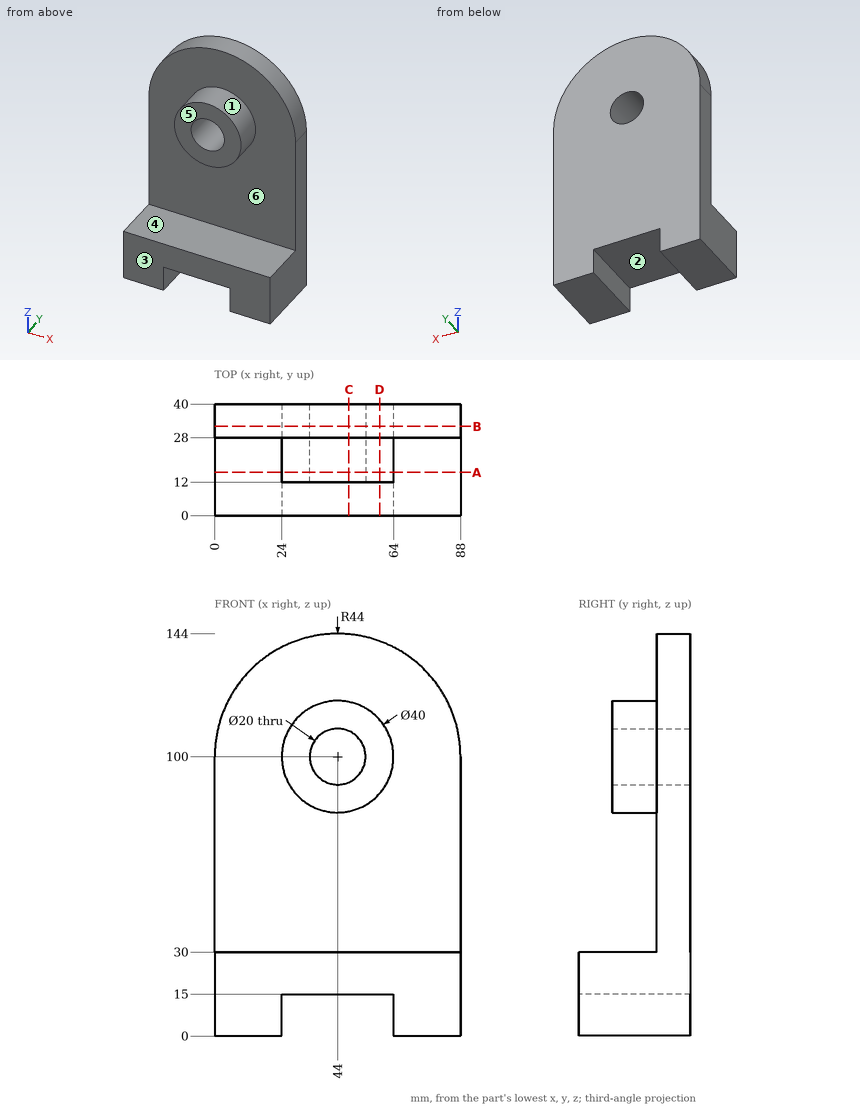
Answer from the drawing. Dimensions are ordinates in mm from the lowest x, y and z of the part. A direction names the side the tool comes from. Round coordinates to 2 decimals unless told otherwise and drop trailing zeros. Write each loop counter-clockwise with the first axis right and the second up, starting at its lowest first coordinate (ties: lowest second). Pieces come first, ordered by that corner, then holes. Notation, with made-up numbers: M 25.5,69.25 L 58.5,69.25 A16 ccw 58.5,85.25 Z; hole C 87,10 d8. An arc over 180 degrees is marked long. One line per item, written item: value.
Q1. Find section D-D on x = 59. Write down the section's boundary in (y, z), plus the area to 3 significant figures.
Data:
outline: M 0,15 L 40,15 L 40,141.36 L 28,141.36 L 28,113.23 L 12,113.23 L 12,86.77 L 28,86.77 L 28,30 L 0,30 Z
area: 2,360 mm2
Q2. Find section C-C on x = 48. Write down the section's boundary in (y, z), plus the area to 3 significant figures.
Data:
outline: M 0,15 L 40,15 L 40,90.83 L 12,90.83 L 12,80.4 L 28,80.4 L 28,30 L 0,30 Z; M 12,109.17 L 40,109.17 L 40,143.82 L 28,143.82 L 28,119.6 L 12,119.6 Z
area: 2,080 mm2
Q3. Which of the six approach directions +Z, -Z, +X, -X, +Y, -Y give full straight-line access (tool end or side, diameter ignored) to the marked faces 4, 5 and 6?
Data:
face 4: +X, -X, -Y
face 5: +Z, +X, -X, -Y
face 6: -Y
Q4. Find section B-B on y = 32. Write down the section's boundary in (x, z).
Data:
outline: M 0,0 L 24,0 L 24,15 L 64,15 L 64,0 L 88,0 L 88,100 A44 ccw 0,100 Z; hole C 44,100 d20
Q5. Straight lines are drawn through the part: line 1 (Z direction, x = 44.5, y = 23); line 2 (Z direction, x = 48.5, y = 12.5); line 3 (Y direction, x = 28.5, z = 63.5). For each, find the intervals that lie inside material, in ascending order. Write a range as [from, to].
Data:
line 1: [15, 30], [80.01, 90.01], [109.99, 119.99]
line 2: [15, 30], [80.51, 91.07], [108.93, 119.49]
line 3: [28, 40]
Q6. Flat-ended cylindrical pins translate along their axes: pin 1 Ø22.5 at (x, y) = (44.5, 17.5) entering from +Z; pin 2 Ø5 at (x, z) = (22, 98.5) entering from -Y; pin 3 Ø12 at (y, z) = (8, 103.5) entering from -X. Find the tip coordinate at first contact, or state that the pin passes through.
Data:
pin 1: z = 144
pin 2: y = 12
pin 3: x = 24
Q7. For a pull along X with two mould halves and no side action, classify the marked faces 1, 2 and 3 as +X half, -X half, draft (parallel to the pull), parting line (faces both ways), or undercut.
Data:
face 1: parting line
face 2: undercut
face 3: draft
Q8. Find section A-A on y = 15.5. Write down the section's boundary in (x, z).
Data:
outline: M 0,0 L 24,0 L 24,15 L 64,15 L 64,0 L 88,0 L 88,30 L 0,30 Z; C 44,100 d40; hole C 44,100 d20
